Part model, mm, in its own coordinate system. Face numbers are marked on the shaded views. A direction names the side the tool comes from. Coordinates: 2 decimals unless noted, no trailing zeros. Loops run counter-clockwise (first coordinate to the right, second up) from the corner with the lowest first, then second, coordinate; pieces in that order, holes last.
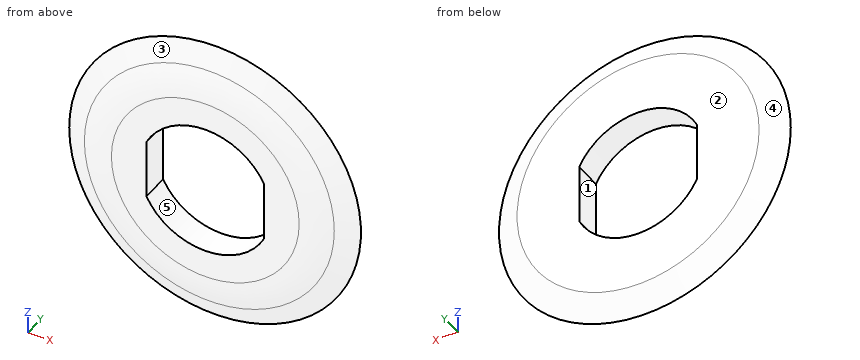
```python
from build123d import *

# Parameters (mm, degrees)
SKETCH2_R           = 9.92
BOSS_EXTRUDE1_DEPTH = 0.96
CUT_EXTRUDE2_DEPTH  = 1.92
FILLET1_R           = 5


with BuildPart() as part:
    # Sketch2 → Boss-Extrude1 (new body, symmetric)
    with BuildSketch(Plane(origin=(0, 0, 0), x_dir=(1, 0, 0), z_dir=(0, 1, 0))):
        Circle(SKETCH2_R)
    extrude(amount=BOSS_EXTRUDE1_DEPTH, both=True)

    # Sketch3 → Cut-Revolve3 (revolve, cut)
    with BuildSketch(Plane.XY):
        Polygon((-9.92, 0.96), (-9.92, 0.171940058), (-8.23, 0.96), align=None)
        Polygon((-7.492546713, -0.96), (-9.92, 0.171940058), (-9.92, -0.96), align=None)
    revolve(axis=Axis((0, 0, 0), (0, 1, 0)), mode=Mode.SUBTRACT)

    # Sketch4 → Cut-Extrude2 (cut)
    with BuildSketch(Plane(origin=(0, 0.96, 0), x_dir=(1, 0, 0), z_dir=(0, 1, 0))):
        with BuildLine():
            Line((4, 0), (4, 2.017523234))
            ThreePointArc((4, 2.017523234), (0, 4.48), (-4, 2.017523234))
            Line((-4, 2.017523234), (-4, 0))
            Line((-4, 0), (-4, -2.017523234))
            ThreePointArc((-4, -2.017523234), (0, -4.48), (4, -2.017523234))
            Line((4, -2.017523234), (4, 0))
        make_face()
    extrude(amount=-CUT_EXTRUDE2_DEPTH, mode=Mode.SUBTRACT)

    # Fillet1
    fillet1_edges = [part.edges().sort_by_distance(p)[0] for p in [
        (7.492546713, -0.96, 0),
    ]]
    fillet(fillet1_edges, radius=FILLET1_R)


solid = part.part
```
Q1. Saw through at A-A (x = 0). List the corners of the cut face in (y, z).
Q2. Saw through at B-B (z = 0). List the corners of the cut face in (x, y), plus the area to 3 significant figures.
Q3. Drop a flat-ended pin along its axis: P1, Ø1, axis at y = 0, z = 0.5, coming from the -X side. Give the stop position or say it passes through.
Q4. Probe line 1 (X direction, y = -0.1, z = 0.5); line 2 (Z direction, x = 1.25, y = 0.6); line 3 (Z direction, x = -3, y = 0.8). List the from-to ranges inside material, lowest first.
Q5. Saw through at C-C (y = 0.45). List the corners of the cut face in (x, z).
Q6. Mould opens along X. For the marked faces 1, 2 and 3 say: released by +X, released by -X, zero draft, split by the parting line, or undercut.
Q7. Tool access for the marked faces 4 and 5: list every direction of +Z, -Z, +X, -X, +Y, -Y with a clear straight run to the whole face (end or side of a thin tool).
Checked values:
1. outline: (-0.96, -6.38) arc R5 ccw to (-0.49, -8.5) - (0.17, -9.92) - (0.96, -8.23) - (0.96, -4.48) - (-0.96, -4.48) - close; (-0.96, 4.48) - (0.96, 4.48) - (0.96, 8.23) - (0.17, 9.92) - (-0.49, 8.5) arc R5 ccw to (-0.96, 6.38) - close
2. outline: (-9.92, 0.17) - (-8.5, -0.49) arc R5 ccw to (-6.38, -0.96) - (-4, -0.96) - (-4, 0.96) - (-8.23, 0.96) - close; (4, -0.96) - (6.38, -0.96) arc R5 ccw to (8.5, -0.49) - (9.92, 0.17) - (8.23, 0.96) - (4, 0.96) - close
2. area: 18.5 mm2
3. P1: stops at x = -9.92
4. line 1: x = -9.32 to -4, 4 to 9.32
4. line 2: z = -8.91 to -4.3, 4.3 to 8.91
4. line 3: z = -8.03 to -3.33, 3.33 to 8.03
5. outline: circle Ø18.65 at (0, 0); hole (-4, -2.02) arc R4.48 ccw to (4, -2.02) - (4, 2.02) arc R4.48 ccw to (-4, 2.02) - close
6. face 1: undercut
6. face 2: zero draft
6. face 3: split by the parting line
7. face 4: +Y
7. face 5: +Y, -Y
